Read the model definition and answer for the solid it produces. Units are mm, in the model's axes. A direction names the side the tool comes from. Coordinates: 2 decimals unless noted, no trailing zeros. Write each loop counter-clockwise with the first axis right and the second up, starting at its lowest first coordinate (ties: lowest second). Pieces come first, ordered by that corner, then holes.
Item 1: Straight lines are drawn through the part: probe 1 along X at (y, z) = (-21.5, 9.5); probe 2 along X at (y, z) = (-13.5, 4.25); probe 3 along X at (y, z) = (-50.5, 2). For each, find the intervals that lie inside material, in ascending order.
Item 2: Section C-C (y = -18) is taken. Give the vertices of the cut face in (x, z), then the cut area to 3 significant figures.
Item 3: A tool of negligible diameter and unlimited length cuts with its end or side. For faces 1 (the face through (17, -10, 5)), 2 (the face through (42, -16.3, -1)), 3 (the face through (24, -59.1, 5)), from which of +Z, -Z, +X, -X, +Y, -Y can it reach the whole face along a straight path? Write none if from no direction.
Item 4: Section A-A (z = 8.5) is taken. Give the vertices of the cut face in (x, y), then the cut area to 3 significant figures.
Item 5: Determine the mould class of faces 4 (the face through (24, -27, 10)), 5 (the face through (10, -18, 3)), 6 (the face through (42, -22, 5)) for opening direction Z: released by +Z, released by -Z, zero draft, split by the parting line, or undercut.
Item 6: Section D-D (x = 24.5) is taken. Give the vertices of the cut face in (y, z).
Item 7: Each of these flat-tipped pins is pushed along its axis until it touches: P1, Ø0.9, axis at x = 16.5, z = 5.5, coming from the +Y side; P2, Ø3.5, axis at x = 24, y = -4.5, coming from the -Z side; P3, Ø0.8, axis at x = 28, z = -1, coming from the -Y side. Where does it stop, or does it pass through?
Item 8: Section B-B (y = -37) is taken. Give the vertices of the cut face in (x, z), then the cut area to 3 significant figures.
from build123d import *

# Parameters (mm, degrees)
SKETCH1_W               = 48
SKETCH1_H               = 70
BOSS_EXTRUDE1_DEPTH     = 10
SKETCH2_R               = 3
CUT_EXTRUDE1_DEPTH      = 86.463442477
SKETCH3_W               = 20.6
SKETCH3_H               = 20.6
CUT_EXTRUDE2_DEPTH      = 86.463442477
FILLET1_R               = 12
SKETCH4_R               = 1.5
CUT_EXTRUDE3_DEPTH      = 86.463442477
SKETCH5_R               = 1.45
CUT_EXTRUDE4_DEPTH      = 10
CUT_EXTRUDE5_DEPTH      = 86.463442477
CUT_EXTRUDE5_DEPTH_BACK = 86.463442477
SKETCH7_W               = 11
SKETCH7_H               = 4.5
SKETCH11_W              = 32
SKETCH11_H              = 15
CUT_EXTRUDE6_DEPTH      = 86.463442477
CUT_EXTRUDE7_DEPTH      = 8
CUT_EXTRUDE7_DEPTH_BACK = 5
SKETCH12_R              = 1.5
SKETCH13_R              = 1.5
BOSS_EXTRUDE4_DEPTH     = 1.6
FILLET2_R               = 8


with BuildPart() as part:
    # Sketch1 → Boss-Extrude1 (new body)
    with BuildSketch(Plane.XY):
        with Locations((24, -35)):
            Rectangle(SKETCH1_W, SKETCH1_H)
    extrude(amount=BOSS_EXTRUDE1_DEPTH)

    # Sketch2 → Cut-Extrude1 (cut, through all)
    with BuildSketch(Plane.XY.offset(10)):
        with Locations((13.5, -13.5)):
            Circle(SKETCH2_R)
        with Locations((34.5, -13.5)):
            Circle(SKETCH2_R)
    extrude(amount=-CUT_EXTRUDE1_DEPTH, mode=Mode.SUBTRACT)

    # Sketch3 → Cut-Extrude2 (cut, through all)
    with BuildSketch(Plane.XY.offset(10)):
        with Locations((24, -48.8)):
            Rectangle(SKETCH3_W, SKETCH3_H)
    extrude(amount=-CUT_EXTRUDE2_DEPTH, mode=Mode.SUBTRACT)

    # Fillet1
    fillet1_edges = [part.edges().sort_by_distance(p)[0] for p in [
        (0, 0, 5),
        (48, 0, 5),
    ]]
    fillet(fillet1_edges, radius=FILLET1_R)

    # Sketch4 → Cut-Extrude3 (cut, through all)
    with BuildSketch(Plane(origin=(0, 0, 0), x_dir=(-1, 0, 0), z_dir=(0, 0, -1))):
        with Locations((-24, -4.5)):
            Circle(SKETCH4_R)
    extrude(amount=-CUT_EXTRUDE3_DEPTH, mode=Mode.SUBTRACT)

    # Sketch5 → Cut-Extrude4 (cut)
    with BuildSketch(Plane(origin=(0, 0, 0), x_dir=(1, 0, 0), z_dir=(0, 1, 0))):
        with Locations(Location((16.5, -5, 0), (0, 0, 270))):
            Circle(SKETCH5_R)
        with Locations(Location((31.5, -5, 0), (0, 0, 270))):
            Circle(SKETCH5_R)
    extrude(amount=-CUT_EXTRUDE4_DEPTH, mode=Mode.SUBTRACT)

    # Sketch7 → Cut-Extrude5 (cut, two sides: drawn at the far end of the back side and taken through both)
    with BuildSketch(Plane(origin=(0, 0, 0), x_dir=(-1, 0, 0), z_dir=(0, 0, -1)).offset(-CUT_EXTRUDE5_DEPTH_BACK)):
        with Locations((-36.5, -21.75)):
            Rectangle(SKETCH7_W, SKETCH7_H)
        with Locations((-11.5, -21.75)):
            Rectangle(SKETCH7_W, SKETCH7_H)
    extrude(amount=CUT_EXTRUDE5_DEPTH + CUT_EXTRUDE5_DEPTH_BACK, mode=Mode.SUBTRACT)

    # Sketch11 → Cut-Extrude6 (cut, through all)
    with BuildSketch(Plane(origin=(0, 0, 0), x_dir=(-1, 0, 0), z_dir=(0, 0, -1))):
        with Locations((-24, -35)):
            Rectangle(SKETCH11_W, SKETCH11_H)
    extrude(amount=-CUT_EXTRUDE6_DEPTH, mode=Mode.SUBTRACT)

    # Sketch12 → Cut-Extrude7 (cut, two sides: drawn at the far end of the back side and taken through both)
    with BuildSketch(Plane(origin=(0, -24, 0), x_dir=(1, 0, 0), z_dir=(0, 1, 0)).offset(-CUT_EXTRUDE7_DEPTH_BACK)):
        with Locations(Location((36.5, -3, 0), (0, 0, 90))):
            Circle(SKETCH12_R)
        with Locations((11.5, -3)):
            Circle(SKETCH12_R)
    extrude(amount=CUT_EXTRUDE7_DEPTH + CUT_EXTRUDE7_DEPTH_BACK, mode=Mode.SUBTRACT)

    # Sketch13 → Boss-Extrude4 (add)
    with BuildSketch(Plane(origin=(0, 0, 0), x_dir=(-1, 0, 0), z_dir=(0, 0, -1))):
        with BuildLine():
            Line((-48, -12), (-48, -16.3))
            Line((-48, -16.3), (-35.577032961, -16.3))
            ThreePointArc((-35.577032961, -16.3), (-36.198367027, -11.027036304), (-31.5, -13.5))
            ThreePointArc((-31.5, -13.5), (-32.027036304, -15.198367027), (-33.422967039, -16.3))
            Line((-33.422967039, -16.3), (-14.577032961, -16.3))
            ThreePointArc((-14.577032961, -16.3), (-15.198367027, -11.027036304), (-10.5, -13.5))
            ThreePointArc((-10.5, -13.5), (-11.027036304, -15.198367027), (-12.422967039, -16.3))
            Line((-12.422967039, -16.3), (0, -16.3))
            Line((0, -16.3), (0, -12))
            ThreePointArc((0, -12), (-3.514718626, -3.514718626), (-12, 0))
            Line((-12, 0), (-36, 0))
            ThreePointArc((-36, 0), (-44.485281374, -3.514718626), (-48, -12))
        make_face()
        with Locations((-24, -4.5)):
            Circle(SKETCH13_R, mode=Mode.SUBTRACT)
    extrude(amount=BOSS_EXTRUDE4_DEPTH)

    # Fillet2
    # the kernel refuses this fillet: 8 mm, written as the material it takes off along each edge
    with BuildSketch(Plane(origin=(13.7, -42.5, -19.155612754), x_dir=(-1, 0, 0), z_dir=(0, 0, 1))) as fillet2_piece_1:
        with BuildLine():
            CenterArc((8, 7.662245102), FILLET2_R, 180, 73.291656284)
            Line((0, 7.662245102), (-0.16, 7.662245102))
            Line((-0.16, 7.662245102), (-0.16, 0))
            Line((-0.16, 0), (0, -0.16))
            ThreePointArc((0, -0.16), (2.85, -0.16), (5.654, -0.153244902))
            Line((5.654, -0.153244902), (5.7, 0))
        make_face()
    extrude(amount=48.311225509, mode=Mode.SUBTRACT)
    with BuildSketch(Plane(origin=(34.3, -42.5, 29.155612754), x_dir=(0, -1, 0), z_dir=(0, 0, -1))) as fillet2_piece_2:
        with BuildLine():
            CenterArc((7.662245102, -8), FILLET2_R, 90, 73.291656284)
            Line((0, -5.7), (-0.153244902, -5.654))
            ThreePointArc((-0.153244902, -5.654), (-0.16, -2.85), (-0.16, 0))
            Line((-0.16, 0), (0, 0.16))
            Line((0, 0.16), (7.662245102, 0.16))
            Line((7.662245102, 0.16), (7.662245102, 0))
        make_face()
    extrude(amount=48.311225509, mode=Mode.SUBTRACT)


solid = part.part
Established:
1. probe 1: x = 0 to 6, 17 to 31, 42 to 48
1. probe 2: x = 0 to 10.5, 16.5 to 31.5, 37.5 to 48
1. probe 3: x = 0 to 13.7, 34.3 to 48
2. outline: (0, 0) - (48, 0) - (48, 10) - (0, 10) - close; hole circle Ø3 at (11.5, 3); hole circle Ø3 at (36.5, 3)
2. area: 466 mm2
3. face 1: +Y
3. face 2: -Z, +X, -X, -Y
3. face 3: +Z, -Z
4. outline: (0, -70) - (48, -70) - (48, -12) arc R12 ccw to (36, 0) - (12, 0) arc R12 ccw to (0, -12) - close; hole (6, -24) - (17, -24) - (17, -19.5) - (6, -19.5) - close; hole (8, -42.5) arc R8 cw to (13.7, -50.16) - (13.7, -59.1) - (34.3, -59.1) - (34.3, -50.16) arc R8 cw to (40, -42.5) - (40, -27.5) - (8, -27.5) - close; hole circle Ø6 at (13.5, -13.5); hole circle Ø3 at (24, -4.5); hole (31, -24) - (42, -24) - (42, -19.5) - (31, -19.5) - close; hole circle Ø6 at (34.5, -13.5)
4. area: 2,290 mm2
5. face 4: released by +Z
5. face 5: undercut
5. face 6: zero draft
6. outline: (-70, 0) - (-59.1, 0) - (-59.1, 10) - (-70, 10) - close; (-27.5, 0) - (-16.3, 0) - (-16.3, -1.6) - (-5.91, -1.6) - (-5.91, 10) - (-27.5, 10) - close; (-3.09, -1.6) - (0, -1.6) - (0, 10) - (-3.09, 10) - close
7. P1: stops at y = -10
7. P2: stops at z = -1.6
7. P3: stops at y = -16.3
8. outline: (0, 0) - (8, 0) - (8, 10) - (0, 10) - close; (40, 0) - (48, 0) - (48, 10) - (40, 10) - close
8. area: 160 mm2
